```python
from build123d import *

# Parameters (mm, degrees)
F0_R      = 19.05
F0_R_2    = 17.4625
F1_DEPTH  = 15.875
F2_DEPTH  = 15.875
F3_R      = 9.525
F4_DEPTH  = 12.7
F5_R      = 18.25625
F5_R_2    = 9.525
F6_DEPTH  = 15.8496
F7_R      = 9.5249999873
F7_R_2    = 9.4615
F8_DEPTH  = 12.7
F9_R      = 2.1618701317
F10_DEPTH = 25.4
F11_R     = 3.81
F11_R_2   = 0.2486890232
F12_DEPTH = 1.524
F13_DEPTH = 2.032
F14_R     = 3.4925
F14_R_2   = 2.54
F15_DEPTH = 9.906
F17_DEPTH = 6.35
F18_R     = 1.5875
F19_DEPTH = 25.4


with BuildPart() as f1:
    # F0 (on Front) → F1 (new body)
    with BuildSketch(Plane.XZ):
        Circle(F0_R)
        Circle(F0_R_2, mode=Mode.SUBTRACT)
    extrude(amount=-F1_DEPTH)

    # F0 (on Front) → F2 (join)
    with BuildSketch(Plane.XZ):
        Circle(F0_R_2)
    extrude(amount=-F2_DEPTH)

    # F3 (on face) → F4 (cut)
    with BuildSketch(Plane.XZ):
        Circle(F3_R)
    extrude(amount=-F4_DEPTH, mode=Mode.SUBTRACT)

    # F5 (on face) → F6 (cut)
    with BuildSketch(Plane(origin=(0, 15.875, 0), x_dir=(-1, 0, 0), z_dir=(0, 1, 0))):
        Circle(F5_R)
        Circle(F5_R_2, mode=Mode.SUBTRACT)
    extrude(amount=-F6_DEPTH, mode=Mode.SUBTRACT)

    # F7 (on face) → F8 (join)
    with BuildSketch(Plane.XZ.offset(-12.7)):
        Circle(F7_R)
        Circle(F7_R_2, mode=Mode.SUBTRACT)
    extrude(amount=F8_DEPTH)

    # F9 (on face) → F10 (cut)
    with BuildSketch(Plane(origin=(0, 15.875, 0), x_dir=(-1, 0, 0), z_dir=(0, 1, 0))):
        with Locations((-4.5284211656, 4.5284211656)):
            Circle(F9_R)
        with Locations((-6.4041546286, 0)):
            Circle(F9_R)
        with Locations((-4.5284211656, -4.5284211656)):
            Circle(F9_R)
        with Locations((0, -6.4041546286)):
            Circle(F9_R)
        with Locations((4.5284211656, -4.5284211656)):
            Circle(F9_R)
        with Locations((6.4041546286, 0)):
            Circle(F9_R)
        with Locations((4.5284211656, 4.5284211656)):
            Circle(F9_R)
        with Locations((0, 6.4041546286)):
            Circle(F9_R)
    extrude(amount=-F10_DEPTH, mode=Mode.SUBTRACT)

    # F11 (on face) → F12 (join)
    with BuildSketch(Plane.XZ.offset(-12.7)):
        Circle(F11_R)
        with Locations((-2.7176439953, -0.8830160614)):
            Circle(F11_R_2, mode=Mode.SUBTRACT)
        with Locations((-1.6795963584, -2.3117660614)):
            Circle(F11_R_2, mode=Mode.SUBTRACT)
        with Locations((0, -2.8575)):
            Circle(F11_R_2, mode=Mode.SUBTRACT)
        with Locations((1.6795963584, -2.3117660614)):
            Circle(F11_R_2, mode=Mode.SUBTRACT)
        with Locations((2.7176439953, -0.8830160614)):
            Circle(F11_R_2, mode=Mode.SUBTRACT)
        with Locations((-2.7176439953, 0.8830160614)):
            Circle(F11_R_2, mode=Mode.SUBTRACT)
        with Locations((-1.6795963584, 2.3117660614)):
            Circle(F11_R_2, mode=Mode.SUBTRACT)
        with BuildLine():
            ThreePointArc((0, 1.905), (1.3470384182, 1.3470384182), (1.905, 0))
            ThreePointArc((1.905, 0), (-1.3470384182, -1.3470384182), (0, 1.905))
        make_face(mode=Mode.SUBTRACT)
        with Locations((1.6795963584, 2.3117660614)):
            Circle(F11_R_2, mode=Mode.SUBTRACT)
        with Locations((2.7176439953, 0.8830160614)):
            Circle(F11_R_2, mode=Mode.SUBTRACT)
        with BuildLine():
            ThreePointArc((0.2486890232, 2.8575), (0.1758496947, 2.6816503053), (0, 2.6088109768))
            ThreePointArc((0, 2.6088109768), (-0.1758496947, 3.0333496947), (0.2486890232, 2.8575))
        make_face(mode=Mode.SUBTRACT)
    extrude(amount=F12_DEPTH)

    # F13 (add): a face of the model
    f13_faces = [f1.faces().sort_by_distance(p)[0] for p in [
        (0, 12.7, 0),
    ]]
    extrude(f13_faces, amount=F13_DEPTH)

    # F14 (on face) → F15 (join)
    with BuildSketch(Plane(origin=(0, 15.875, 0), x_dir=(-1, 0, 0), z_dir=(0, 1, 0))):
        Circle(F14_R)
        Circle(F14_R_2, mode=Mode.SUBTRACT)
    extrude(amount=F15_DEPTH)

    # F16 (on face) → F17 (join)
    with BuildSketch(Plane(origin=(0, 0.0254, 0), x_dir=(-1, 0, 0), z_dir=(0, 1, 0))):
        with BuildLine():
            ThreePointArc((-0.1918367084, 9.5230679761), (-0.0959232185, 9.5245169818), (0, 9.525))
            ThreePointArc((0, 9.525), (0.1051390114, 9.5244197087), (0.210265212, 9.5226789057))
            Line((0.210265212, 9.5226789057), (0.210265212, 13.3574450496))
            ThreePointArc((0.210265212, 13.3574450496), (0.5715, 13.8888590037), (0.210265212, 14.4202729578))
            Line((0.210265212, 14.4202729578), (0.210265212, 18.2550391017))
            ThreePointArc((0.210265212, 18.2550391017), (0.0092148106, 18.2562476744), (-0.1918367084, 18.2552420619))
            Line((-0.1918367084, 18.2552420619), (-0.1918367084, 14.4271999062))
            ThreePointArc((-0.1918367084, 14.4271999062), (-0.5715, 13.8888590037), (-0.1918367084, 13.3505181011))
            Line((-0.1918367084, 13.3505181011), (-0.1918367084, 9.5230679761))
        make_face()
        with BuildLine():
            ThreePointArc((-8.3431371434, 4.5953985252), (-8.244279957, 4.770479325), (-8.1417492384, 4.943434468))
            Line((-8.1417492384, 4.943434468), (-11.4627541366, 6.8608175399))
            ThreePointArc((-11.4627541366, 6.8608175399), (-11.7423547268, 7.4393630201), (-12.383190105, 7.392231494))
            Line((-12.383190105, 7.392231494), (-15.7041950031, 9.3096145659))
            ThreePointArc((-15.7041950031, 9.3096145659), (-15.8057668585, 9.1361040973), (-15.905421732, 8.9614855682))
            Line((-15.905421732, 8.9614855682), (-12.5902399784, 7.0474644903))
            ThreePointArc((-12.5902399784, 7.0474644903), (-12.3138547268, 6.4494959836), (-11.6578061835, 6.5091235878))
            Line((-11.6578061835, 6.5091235878), (-8.3431371434, 4.5953985252))
        make_face()
        with BuildLine():
            ThreePointArc((-8.1513004351, -4.9276694509), (-8.2534962622, -4.7545162162), (-8.3520144504, -4.5792444377))
            Line((-8.3520144504, -4.5792444377), (-11.6730193486, -6.4966275097))
            ThreePointArc((-11.6730193486, -6.4966275097), (-12.3138547268, -6.4494959836), (-12.5934553169, -7.0280414638))
            Line((-12.5934553169, -7.0280414638), (-15.9144602151, -8.9454245357))
            ThreePointArc((-15.9144602151, -8.9454245357), (-15.8149816691, -9.1201435771), (-15.7135850237, -9.2937564938))
            Line((-15.7135850237, -9.2937564938), (-12.3984032701, -7.3797354159))
            ThreePointArc((-12.3984032701, -7.3797354159), (-11.7423547268, -7.4393630201), (-11.4659694751, -6.8413945134))
            Line((-11.4659694751, -6.8413945134), (-8.1513004351, -4.9276694509))
        make_face()
        with BuildLine():
            ThreePointArc((0.1918367084, -9.5230679761), (-0.0092163051, -9.5249955412), (-0.210265212, -9.5226789057))
            Line((-0.210265212, -9.5226789057), (-0.210265212, -13.3574450496))
            ThreePointArc((-0.210265212, -13.3574450496), (-0.5715, -13.8888590037), (-0.210265212, -14.4202729578))
            Line((-0.210265212, -14.4202729578), (-0.210265212, -18.2550391017))
            ThreePointArc((-0.210265212, -18.2550391017), (-0.0092148106, -18.2562476744), (0.1918367084, -18.2552420619))
            Line((0.1918367084, -18.2552420619), (0.1918367084, -14.4271999062))
            ThreePointArc((0.1918367084, -14.4271999062), (0.5715, -13.8888590037), (0.1918367084, -13.3505181011))
            Line((0.1918367084, -13.3505181011), (0.1918367084, -9.5230679761))
        make_face()
        with BuildLine():
            Line((11.6578061835, -6.5091235878), (8.3431371434, -4.5953985252))
            ThreePointArc((8.3431371434, -4.5953985252), (8.244279957, -4.770479325), (8.1417492384, -4.943434468))
            Line((8.1417492384, -4.943434468), (11.4627541366, -6.8608175399))
            ThreePointArc((11.4627541366, -6.8608175399), (11.7423547268, -7.4393630201), (12.383190105, -7.392231494))
            Line((12.383190105, -7.392231494), (15.7041950031, -9.3096145659))
            ThreePointArc((15.7041950031, -9.3096145659), (15.8057668585, -9.1361040973), (15.905421732, -8.9614855682))
            Line((15.905421732, -8.9614855682), (12.5902399784, -7.0474644903))
            ThreePointArc((12.5902399784, -7.0474644903), (12.3138547268, -6.4494959836), (11.6578061835, -6.5091235878))
        make_face()
        with BuildLine():
            Line((11.4659694751, 6.8413945134), (8.1513004351, 4.9276694509))
            ThreePointArc((8.1513004351, 4.9276694509), (8.2534962622, 4.7545162162), (8.3520144504, 4.5792444377))
            Line((8.3520144504, 4.5792444377), (11.6730193486, 6.4966275097))
            ThreePointArc((11.6730193486, 6.4966275097), (12.3138547268, 6.4494959836), (12.5934553169, 7.0280414638))
            Line((12.5934553169, 7.0280414638), (15.9144602151, 8.9454245357))
            ThreePointArc((15.9144602151, 8.9454245357), (15.8149816691, 9.1201435771), (15.7135850237, 9.2937564938))
            Line((15.7135850237, 9.2937564938), (12.3984032701, 7.3797354159))
            ThreePointArc((12.3984032701, 7.3797354159), (11.7423547268, 7.4393630201), (11.4659694751, 6.8413945134))
        make_face()
    extrude(amount=F17_DEPTH)

    # F18 (on face) → F19 (cut)
    with BuildSketch(Plane.XZ.offset(-10.668)):
        Circle(F18_R)
    extrude(amount=-F19_DEPTH, mode=Mode.SUBTRACT)


solid = f1.part
```
CAD build for the part. Positions are in the model's coordinates, mm. A direction names the side the tool comes from. Coordinates: 2 decimals unless noted, no trailing zeros. Write each loop counter-clockwise with the first axis right and the second up, starting at its lowest first coordinate (ties: lowest second). Pieces come first, ordered by that corner, then holes. Notation, with made-up numbers: (-32.5, -35) -> (24.5, -35) arc R11 ccw to (24.5, -22) -> close; hole circle Ø10 at (8, 46.25). An arc over 180 degrees is marked (long way). Return JSON: item names as keys, results as strings. Group by question number.
Q1. Cut at A-A, the plane y = 14.75. State how many separate pieces and enclosed holes the cut face has, then the cut area to 3 significant figures.
Q2. Flat gauge pins, fed straight in: pin 1 (3 mm diameter, centred on y = 3.5, z = 15.5, fed in from -X); pin 2 (1.2 mm diameter, centred on y = 3.5, z = -11.5, fed in from +X); pin 3 (2 mm diameter, centred on y = 7, z = -6.5, fed in from -X); pin 4 (2.5 mm diameter, centred on x = 4.53, z = 4.53, fed in from -Y). Where does each tip first touch, or does it go through?
Q3. Cut at C-C, the plane y = 18. Give the cut face in (x, z) (1 decimal).
Q4. Which spindle directions (+Z, -Z, +X, -X, +Y, -Y) get a long thin tool onto all of the face, cutting with end or side? Do faces 3 (the face through (4, 12.7, 0)), 4 (the face through (2.466, 14.31, -3.879)), 5 (the face through (-14.08, 3.16, 8.35)). Say none if no direction does.
Q5. Drill centre lines: line 1 (Z direction, x = 0, y = 20.75); line 2 (X direction, y = 1.5, z = 11.5); line 3 (X direction, y = 1.5, z = -16.5). Where is each one in solid material? Low to high.
Q6. Pull direction X, two halves, no side cores. Call faces 1 (the face through (0.33, 20.76, 2.52)), 2 (the face through (-15.12, 7.83, -11.59)): released by +X, released by -X, zero draft, split by the parting line, or undercut.
Q7. Cut at B-B, the plane z = -15.5. Give the cut face in (x, y) (3 decimals), then the cut area to 3 significant figures.
Returned:
{
 "1": {"separate pieces": "2", "enclosed holes": "10", "area": "253 mm2"},
 "2": {"pin 1": "stops at x = -12.92", "pin 2": "stops at x = 15.62", "pin 3": "stops at x = -18.24", "pin 4": "passes through"},
 "3": {"outline": "circle Ø7 at (0, 0); hole circle Ø5.1 at (0, 0)"},
 "4": {"face 3": "-Y", "face 4": "+Y, -Y", "face 5": "+Y"},
 "5": {"line 1": "z = -3.49 to -2.54, 2.54 to 3.49", "line 2": "x = -15.19 to -14.18, -0.21 to 0.19, 14.18 to 15.19", "line 3": "x = -9.52 to -7.81, -0.19 to 0.21, 7.81 to 9.52"},
 "6": {"face 1": "undercut", "face 2": "split by the parting line"},
 "7": {"outline": "(-11.075, 0) -> (11.075, 0) -> (11.075, 15.875) -> (9.646, 15.875) -> (9.646, 0.025) -> (0.21, 0.025) -> (0.21, 6.375) -> (-0.192, 6.375) -> (-0.192, 0.025) -> (-9.646, 0.025) -> (-9.646, 15.875) -> (-11.075, 15.875) -> close", "area": "48.4 mm2"}
}
